CAD build for the part. Positions are in the model's coordinates, mm. Face numbers are marked on the shaded views. A direction names the side the tool comes from. Round coordinates to 2 decimals unless told otherwise and drop trailing zeros. Loops run counter-clockwise (first coordinate to the right, second up) from the corner with the lowest first, then second, coordinate; pieces in that order, holes last. Notation, with made-up numbers: (57, 83) - (65, 83) arc R17 ccw to (65, 108) - close; hole circle Ø10 at (41.5, 46.5). An arc over 180 degrees is marked (long way). Use one line per item in the form item = value.
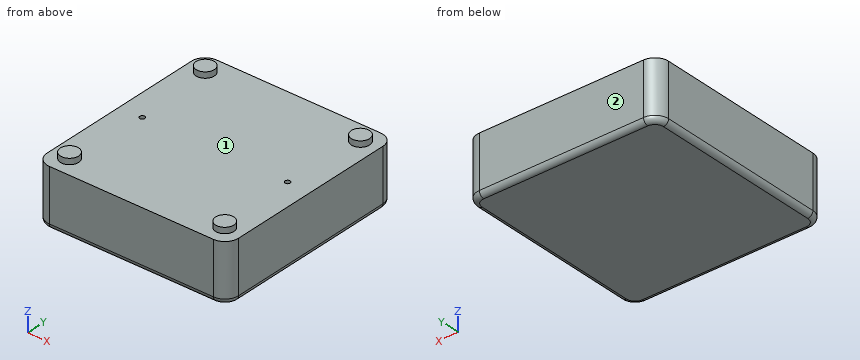
from build123d import *

# Parameters (mm, degrees)
SKETCH_1_W          = 112
SKETCH_1_H          = 117
EXTRUDE_1_DEPTH     = 33.5
FILLET_1_R          = 8
SKETCH_2_R          = 1.5
CUT_EXTRUDE_1_DEPTH = 3
SKETCH_3_R          = 5.35
EXTRUDE_2_DEPTH     = 3.4
FILLET_2_R          = 3


with BuildPart() as part:
    # 草图1 → 凸台-拉伸1 (new body)
    with BuildSketch(Plane.XY):
        with Locations((-117.832945126, 6.678161232)):
            Rectangle(SKETCH_1_W, SKETCH_1_H)
    extrude(amount=EXTRUDE_1_DEPTH)

    # 圆角1
    fillet_1_edges = [part.edges().sort_by_distance(p)[0] for p in [
        (-173.832945126, 65.178161232, 16.75),
        (-61.832945126, 65.178161232, 16.75),
        (-61.832945126, -51.821838768, 16.75),
        (-173.832945126, -51.821838768, 16.75),
    ]]
    fillet(fillet_1_edges, radius=FILLET_1_R)

    # 草图2 → 切除-拉伸1 (cut)
    with BuildSketch(Plane.XY.offset(33.5)):
        with Locations((-75.332945126, 6.678161232)):
            Circle(SKETCH_2_R)
        with Locations((-160.332945126, 6.678161232)):
            Circle(SKETCH_2_R)
    extrude(amount=-CUT_EXTRUDE_1_DEPTH, mode=Mode.SUBTRACT)

    # 草图3 → 凸台-拉伸2 (add)
    with BuildSketch(Plane.XY.offset(33.5)):
        with Locations((-72.432945126, -40.821838768)):
            Circle(SKETCH_3_R)
        with Locations((-163.232945126, -40.821838768)):
            Circle(SKETCH_3_R)
        with Locations((-163.232945126, 54.178161232)):
            Circle(SKETCH_3_R)
        with Locations((-72.432945126, 54.178161232)):
            Circle(SKETCH_3_R)
    extrude(amount=EXTRUDE_2_DEPTH)

    # 圆角2
    fillet_2_edges = [part.edges().sort_by_distance(p)[0] for p in [
        (-117.832945126, 65.178161232, 0),
        (-173.832945126, 6.678161232, 0),
        (-61.832945126, 6.678161232, 0),
        (-117.832945126, -51.821838768, 0),
        (-64.176090876, -49.478693018, 0),
        (-171.489799375, -49.478693018, 0),
        (-171.489799375, 62.835015481, 0),
        (-64.176090876, 62.835015481, 0),
    ]]
    fillet(fillet_2_edges, radius=FILLET_2_R)


solid = part.part
1) Slice it at B-B (x = -130.5). Write the cut outline in (y, z), plus the area to 3 significant figures.
Report:
outline = (-51.82, 3) arc R3 ccw to (-48.82, 0) - (62.18, 0) arc R3 ccw to (65.18, 3) - (65.18, 33.5) - (-51.82, 33.5) - close
area = 3,920 mm^2
2) Slice it at A-A (y = -32). Write the cut outline in (x, z).
Report:
outline = (-173.83, 3) arc R3 ccw to (-170.83, 0) - (-64.83, 0) arc R3 ccw to (-61.83, 3) - (-61.83, 33.5) - (-173.83, 33.5) - close
3) Drill centre lines: probe 1 along Z at (x, y) = (-126, 15); probe 2 along Y at (x, z) = (-167, 18); probe 3 along X at (y, z) = (-37, 2.5). Where is each one in solid material? Low to high.
Report:
probe_1 = 0 to 33.5
probe_2 = -51.74 to 65.09
probe_3 = -173.79 to -61.87
4) Flat gauge pins, fed straight in: pin 1 (1 mm diameter, centred on x = -147, y = 50.5, fed in from +Z); pin 2 (0.9 mm diameter, centred on x = -161, y = 7, fed in from +Z). Where does each tip first touch, or does it go through?
Report:
pin_1 = 33.5
pin_2 = 30.5
5) Tool access for the marked faces 1 and 2: list every direction of +Z, -Z, +X, -X, +Y, -Y with a clear straight run to the whole face (end or side of a thin tool).
Report:
face_1 = +Z
face_2 = +Z, -Z, +X, -X, +Y
